Autodesk Inventor part; units mm, degrees
ref_plane "YZ Plane" through (0, 0, 0) normal (1, 0, 0) x (0, 1, 0)
ref_plane "XZ Plane" through (0, 0, 0) normal (0, 1, 0) x (-1, 0, 0)
ref_plane "XY Plane" through (0, 0, 0) normal (0, 0, 1) x (1, 0, 0)
sketch "Sketch1" plane through (0, 0, 0) normal (0, 1, 0) x (-1, 0, 0)
  line L0 (7, 10) -> (-7, 10)
  line L1 (-7, 10) -> (-7, -10)
  line L2 (-7, -10) -> (7, -10)
  line L3 (7, -10) -> (7, 10)
  line L4 (7, 10) -> (-7, -10) construction
  line L5 (-7, 10) -> (7, -10) construction
  point P0 (0, 0)
  dimension "POST_WIDTH" = 20
  dimension "POST_LENGTH" = 14
extrude "Extrusion1" add sketch "Sketch1" along normal blind 5.075
sketch "Sketch2" plane through (0, 0, 0) normal (0, -1, 0) x (1, 0, 0)
  line L0 (-7, -19) -> (7, -19)
  line L1 (7, -19) -> (7, 19)
  line L2 (7, 19) -> (-7, 19)
  line L3 (-7, 19) -> (-7, -19)
  line L4 (-7, -19) -> (7, 19) construction
  line L5 (7, -19) -> (-7, 19) construction
  line L6 (-7, -10) -> (-7, 10)
  line L7 (-7, 10) -> (7, 10)
  point P0 (0, 0)
  dimension "d4" = 0
  dimension "WING_LENGTH" = 9
extrude "Extrusion2" add sketch "Sketch2" against normal blind 5.075
sketch "Sketch3" plane through (0, 5.075, 0) normal (0, 1, 0) x (1, 0, 0)
  line L0 (-7, 19) -> (7, 19)
  line L1 (0, 19) -> (0, -19)
  line L2 (7, -19) -> (-7, -19)
  line L3 (7, 0) -> (-7, 0)
  line L4 (-7, -19) -> (-7, 19)
  point P0 (0, 0)
  point P1 (0, -13)
  point P2 (0, 13)
  dimension "d15" = 0
  dimension "d16" = 6
hole "Hole1" at (0, 5.075, 13) at (0, 5.075, -13) direction (0, -1, 0) diameter 4.5 end through all counterbore diameter 8 counterbore depth 2.075
chamfer "Chamfer4" distance 1 angle 45 4 edges at (-7, 2.5375, 19) (7, 2.5375, 19) (-7, 2.5375, -19) (7, 2.5375, -19)
sketch "Sketch4" plane through (0, 5.075, 0) normal (0, 1, 0) x (1, 0, 0)
  line L0 (7, 10) -> (5, 10)
  line L1 (5, 10) -> (5, -10)
  line L2 (5, -10) -> (7, -10)
  line L3 (7, -10) -> (7, 10)
  line L4 (7, -18) -> (7, 18)
  point P0 (0, 0)
  dimension "d56" = 20
  dimension "d57" = 2
  dimension "d58" = 0
  dimension "d59" = 10
extrude "Extrusion3" add sketch "Sketch4" along normal blind 2
sketch "Sketch5" plane through (0, 0, 0) normal (0, -1, 0) x (1, 0, 0)
  line L0 (-9.8, 0) -> (9.8, 0)
  line L1 (0, 26.6) -> (0, -26.6)
  line L2 (-7, 19) -> (-7, -19)
  line L3 (7, -10) -> (7, -18)
  line L4 (6, -19) -> (7, -18)
  line L5 (6, -19) -> (-6, -19)
  line L6 (-7, -18) -> (-6, -19)
  line L7 (-7, -18) -> (-7, 18)
  line L8 (-6, 19) -> (-7, 18)
  line L9 (-6, 19) -> (6, 19)
  line L10 (7, 18) -> (6, 19)
  line L11 (5, -10) -> (7, -10)
  line L12 (7, 18) -> (7, 10)
  line L13 (7, 10) -> (5, 10)
  line L14 (5, 10) -> (5, -10)
  point P0 (-0.5, 0)
hole "Hole2" at (-0.5, 0, 0) direction (0, 1, 0) diameter 4.5 end through all
chamfer "Chamfer1" distance 1 angle 45 2 edges at (6, 7.075, -10) (6, 7.075, 10)
chamfer "Chamfer2" [suppressed]
sketch "Sketch7" plane through (0, 5.075, 0) normal (0, 1, 0) x (1, 0, 0)
  circle A0 centre (-0.5, 0) radius 2.75
  circle A1 centre (-0.5, 0) radius 2.25
  point P0 (0, 0)
  dimension "d46" = 5.5
extrude "Extrusion5" cut sketch "Sketch7" against normal blind 0.5 contours A0 | A1
equation "\"POST_LENGTH\" = 2 * LIP_THICKNESS + BASE_THICKNESS"
equation "\"POST_HEIGHT\" = BEAM_HEIGHT - BASE2APERTURE_CENTER"
equation "\"BASE2APERTURE_CENTER\" = 13.975"
equation "\"BEAM_HEIGHT\" = 19.05"
equation "\"WALL_GAP\" = 0.5"
properties part number "ADAPTER_RSP05-BH19.05"
The model under review builds one solid part; all positions refer to its coordinate system, in mm. A direction names the side the tool comes from. Give positions to 0.01 mm unless a question says otherwise; leave off trailing zeros. Order: outer loops, then holes, each group sorted by start corner. A loop starts at its lowest first (then second) coordinate and runs counter-clockwise, first axis right, second up. Notation, with made-up numbers: M -27.75,66.25 L 14.25,66.25 A26 ccw 14.25,90.25 Z; hole C 43.5,64.5 d1. An arc over 180 degrees is marked long. Answer in a Markdown table with one row per item. Add a question column.
1. To check wall thickness, follow line 1 along X through (y, z) = (3.5, -13); line 2 along Z through (x, y) = (2.5, 4.25); line 3 along Z through (x, y) = (0, 1.9). State the ranges of each line that lie inside material, in increasing order.
2. Add section B-B on x = -0.5. State the section outline as (y, z) points (3 decimals), plus the area to 3 significant figures.
3. For pin 1 Ø2.5 at (x, z) = (-2, 13.5) entering from +Y; pin 2 Ø1.1 at (x, y) = (6.5, 5.5) entering from +Z; pin 3 Ø6 at (x, z) = (0, -0.5) entering from +Y (3 decimals), all flat-tipped, find the tip position at first contact; note any pin that passes through.
4. Add section A-A on z = 0. State the section outline as (x, y) points (3 decimals).
5. Add section C-C on z = 13. State the section outline as (x, y) points (3 decimals), plus the area to 4 significant figures.
6. Mouldability with a two-part tool opening along X and no side actions: class faces 1 (the flat face through (6.5, 2.6, 18.5)), 2 (the flat face through (2, 3, -11)), 3 (the flat face through (5, 6, 0)) as released by +X, released by -X, zero draft, split by the parting line, or undercut.
7. Machinability: for faces 4 (the flat face through (6, 5.6, -10)), 5 (the cylindrical face through (0.869, 2.32, 1.786)), 6 (the flat face through (6, 5.6, 10)), 7 (the flat face through (6, 7.075, 0)), 8 (the cylindrical face through (2.4, 4, 9.8)), which of the approach directions +Z, -Z, +X, -X, +Y, -Y give a long, thin tool a straight path to every point of the face, cutting with its end or side? Answer none if there is none.
8. Add section D-D on x = 3. State the section outline as (y, z) points (3 decimals), plus the area to 3 significant figures.
The answers:
| question | item | result |
|---|---|---|
| 1 | line 1 | -7 to -4, 4 to 7 |
| 1 | line 2 | -19 to -16.12, -9.88 to 9.88, 16.12 to 19 |
| 1 | line 3 | -19 to -15.25, -10.75 to -2.19, 2.19 to 10.75, 15.25 to 19 |
| 2 | outline | M 0,-19 L 5.075,-19 L 5.075,-16.969 L 3,-16.969 L 3,-15.194 L 0,-15.194 Z; M 0,-10.806 L 3,-10.806 L 3,-9.031 L 5.075,-9.031 L 5.075,-2.75 L 4.575,-2.75 L 4.575,-2.25 L 0,-2.25 Z; M 0,2.25 L 4.575,2.25 L 4.575,2.75 L 5.075,2.75 L 5.075,9.031 L 3,9.031 L 3,10.806 L 0,10.806 Z; M 0,15.194 L 3,15.194 L 3,16.969 L 5.075,16.969 L 5.075,19 L 0,19 Z |
| 2 | area | 110 mm2 |
| 3 | pin 1 | y = 3 |
| 3 | pin 2 | z = 18.85 |
| 3 | pin 3 | y = 5.075 |
| 4 | outline | M -7,0 L -2.75,0 L -2.75,4.575 L -3.25,4.575 L -3.25,5.075 L -7,5.075 Z; M 1.75,0 L 7,0 L 7,7.075 L 5,7.075 L 5,5.075 L 2.25,5.075 L 2.25,4.575 L 1.75,4.575 Z |
| 5 | outline | M -7,0 L -2.25,0 L -2.25,3 L -4,3 L -4,5.075 L -7,5.075 Z; M 2.25,0 L 7,0 L 7,5.075 L 4,5.075 L 4,3 L 2.25,3 Z |
| 5 | area | 40.95 mm2 |
| 6 | face 1 | released by +X |
| 6 | face 2 | undercut |
| 6 | face 3 | released by -X |
| 7 | face 4 | -Z, +X, -X, +Y |
| 7 | face 5 | +Y, -Y |
| 7 | face 6 | +Z, +X, -X, +Y |
| 7 | face 7 | +Z, -Z, +X, -X, +Y |
| 7 | face 8 | +Y |
| 8 | outline | M 0,-19 L 5.075,-19 L 5.075,-15.646 L 3,-15.646 L 3,-10.354 L 5.075,-10.354 L 5.075,10.354 L 3,10.354 L 3,15.646 L 5.075,15.646 L 5.075,19 L 0,19 Z |
| 8 | area | 171 mm2 |
